Could you check a few things on this model? Use its own coordinates, in mm. A direction names the side the tool comes from. Coordinates: 2 decimals unless noted, no trailing zeros. Write each loop counter-clockwise with the first axis right and the second up, starting at its lowest first coordinate (ties: lowest second). Pieces come first, ordered by that corner, then holes. Notation, with made-up numbers: M 47.5,13 L 84.5,13 A19 cw 84.5,41 Z; hole C 81.25,-7 d3. An arc over 180 degrees is marked long. Write item = value, one per line.
```python
from build123d import *

# Parameters (mm, degrees)
ESBO_O1_W                = 100
ESBO_O1_H                = 95
RESSALTO_EXTRUS_O1_DEPTH = 1.5
ESBO_O2_R                = 1.5
ESBO_O2_W                = 40
ESBO_O2_H                = 3
CORTE_EXTRUS_O1_DEPTH    = 4
ESBO_O3_W                = 3
ESBO_O3_H                = 32
RESSALTO_EXTRUS_O2_DEPTH = 3
CUT_EXTRUDE1_DEPTH       = 1
CUT_EXTRUDE1_DEPTH_BACK  = 4
CUT_EXTRUDE4_DEPTH       = 2.5
CUT_EXTRUDE4_DEPTH_BACK  = 2.5
FILLET1_R                = 5
SKETCH3_W                = 3
SKETCH3_H                = 30
SKETCH3_H_2              = 17
SKETCH3_W_2              = 8
SKETCH3_H_3              = 3
CUT_EXTRUDE5_DEPTH       = 2.5
CUT_EXTRUDE5_DEPTH_BACK  = 2.5
SKETCH4_R                = 1.1
SKETCH4_W                = 12.2
SKETCH4_H                = 22.5
CUT_EXTRUDE6_DEPTH       = 1
CUT_EXTRUDE6_DEPTH_BACK  = 4


with BuildPart() as part:
    # Esboço1 → Ressalto-extrusão1 (new body, symmetric)
    with BuildSketch(Plane.XY):
        Rectangle(ESBO_O1_W, ESBO_O1_H)
    extrude(amount=RESSALTO_EXTRUS_O1_DEPTH, both=True)

    # Esboço2 → Corte-extrusão1 (cut, through all)
    with BuildSketch(Plane.XY.offset(1.5)):
        with Locations((-33, -1)):
            Circle(ESBO_O2_R)
        with Locations((33, -1)):
            Circle(ESBO_O2_R)
        with Locations((0, -46)):
            Rectangle(ESBO_O2_W, ESBO_O2_H)
        with Locations((0, -1)):
            Rectangle(ESBO_O2_W, ESBO_O2_H)
    extrude(amount=-CORTE_EXTRUS_O1_DEPTH, mode=Mode.SUBTRACT)

    # Esboço3 → Ressalto-extrusão2 (add, through all)
    with BuildSketch(Plane.XY.offset(1.5)):
        with Locations((-51.5, -31.5)):
            Rectangle(ESBO_O3_W, ESBO_O3_H)
        with Locations((51.5, -31.5)):
            Rectangle(ESBO_O3_W, ESBO_O3_H)
        with Locations((-51.5, 31.5)):
            Rectangle(ESBO_O3_W, ESBO_O3_H)
        with Locations((51.5, 31.5)):
            Rectangle(ESBO_O3_W, ESBO_O3_H)
    extrude(amount=-RESSALTO_EXTRUS_O2_DEPTH)

    # Sketch1 → Cut-Extrude1 (cut, two sides)
    with BuildSketch(Plane(origin=(0, 0, -1.5), x_dir=(-1, 0, 0), z_dir=(0, 0, -1))) as cut_extrude1_sk:
        with BuildLine():
            Line((-36.5, 39.75), (-36.5, 26.75))
            ThreePointArc((-36.5, 26.75), (-36.939339828, 25.689339828), (-38, 25.25))
            Line((-38, 25.25), (-41, 25.25))
            ThreePointArc((-41, 25.25), (-42.060660172, 24.810660172), (-42.5, 23.75))
            Line((-42.5, 23.75), (-42.5, 23.5))
            ThreePointArc((-42.5, 23.5), (-44, 22), (-45.5, 23.5))
            Line((-45.5, 23.5), (-45.5, 23.75))
            ThreePointArc((-45.5, 23.75), (-45.74500996, 24.571583836), (-46.4, 25.124772708))
            ThreePointArc((-46.4, 25.124772708), (-46.836660027, 25.49356529), (-47, 26.041287847))
            Line((-47, 26.041287847), (-47, 40.458712153))
            ThreePointArc((-47, 40.458712153), (-46.836660027, 41.00643471), (-46.4, 41.375227292))
            ThreePointArc((-46.4, 41.375227292), (-45.74500996, 41.928416164), (-45.5, 42.75))
            Line((-45.5, 42.75), (-45.5, 43))
            ThreePointArc((-45.5, 43), (-44, 44.5), (-42.5, 43))
            Line((-42.5, 43), (-42.5, 42.75))
            ThreePointArc((-42.5, 42.75), (-42.060660172, 41.689339828), (-41, 41.25))
            Line((-41, 41.25), (-38, 41.25))
            ThreePointArc((-38, 41.25), (-36.939339828, 40.810660172), (-36.5, 39.75))
        make_face()
        with BuildLine():
            Line((47, 40.458712153), (47, 26.041287847))
            ThreePointArc((47, 26.041287847), (46.836660027, 25.49356529), (46.4, 25.124772708))
            ThreePointArc((46.4, 25.124772708), (45.74500996, 24.571583836), (45.5, 23.75))
            Line((45.5, 23.75), (45.5, 23.5))
            ThreePointArc((45.5, 23.5), (44, 22), (42.5, 23.5))
            Line((42.5, 23.5), (42.5, 23.75))
            ThreePointArc((42.5, 23.75), (42.060660172, 24.810660172), (41, 25.25))
            Line((41, 25.25), (38, 25.25))
            ThreePointArc((38, 25.25), (36.939339828, 25.689339828), (36.5, 26.75))
            Line((36.5, 26.75), (36.5, 39.75))
            ThreePointArc((36.5, 39.75), (36.939339828, 40.810660172), (38, 41.25))
            Line((38, 41.25), (41, 41.25))
            ThreePointArc((41, 41.25), (42.060660172, 41.689339828), (42.5, 42.75))
            Line((42.5, 42.75), (42.5, 43))
            ThreePointArc((42.5, 43), (44, 44.5), (45.5, 43))
            Line((45.5, 43), (45.5, 42.75))
            ThreePointArc((45.5, 42.75), (45.74500996, 41.928416164), (46.4, 41.375227292))
            ThreePointArc((46.4, 41.375227292), (46.836660027, 41.00643471), (47, 40.458712153))
        make_face()
    extrude(amount=CUT_EXTRUDE1_DEPTH, mode=Mode.SUBTRACT)
    extrude(cut_extrude1_sk.sketch, amount=-CUT_EXTRUDE1_DEPTH_BACK, mode=Mode.SUBTRACT)

    # Sketch2 → Cut-Extrude4 (cut, two sides)
    with BuildSketch(Plane.XY) as cut_extrude4_sk:
        with BuildLine():
            Line((-0.5, -32.5), (0.5, -32.5))
            ThreePointArc((0.5, -32.5), (1.207106781, -32.792893219), (1.5, -33.5))
            Line((1.5, -33.5), (1.5, -38.23))
            Line((1.5, -38.23), (2.85, -38.23))
            Line((2.85, -38.23), (2.85, -40.5))
            Line((2.85, -40.5), (1.5, -40.5))
            Line((1.5, -40.5), (1.5, -44.5))
            Line((1.5, -44.5), (-1.5, -44.5))
            Line((-1.5, -44.5), (-1.5, -40.5))
            Line((-1.5, -40.5), (-2.85, -40.5))
            Line((-2.85, -40.5), (-2.85, -38.23))
            Line((-2.85, -38.23), (-1.5, -38.23))
            Line((-1.5, -38.23), (-1.5, -33.5))
            ThreePointArc((-1.5, -33.5), (-1.207106781, -32.792893219), (-0.5, -32.5))
        make_face()
    extrude(amount=CUT_EXTRUDE4_DEPTH, mode=Mode.SUBTRACT)
    extrude(cut_extrude4_sk.sketch, amount=-CUT_EXTRUDE4_DEPTH_BACK, mode=Mode.SUBTRACT)

    # Fillet1
    fillet1_edges = [part.edges().sort_by_distance(p)[0] for p in [
        (53, 47.5, 0),
        (-53, 47.5, 0),
    ]]
    fillet(fillet1_edges, radius=FILLET1_R)

    # Sketch3 → Cut-Extrude5 (cut, two sides)
    with BuildSketch(Plane.XY) as cut_extrude5_sk:
        with Locations((7.5, 29.5)):
            Rectangle(SKETCH3_W, SKETCH3_H)
        with Locations((7.5, -17)):
            Rectangle(SKETCH3_W, SKETCH3_H_2)
        with Locations((-7.5, 29.5)):
            Rectangle(SKETCH3_W, SKETCH3_H)
        with Locations((-1.5, -24)):
            Rectangle(SKETCH3_W_2, SKETCH3_H_3)
    extrude(amount=CUT_EXTRUDE5_DEPTH, mode=Mode.SUBTRACT)
    extrude(cut_extrude5_sk.sketch, amount=-CUT_EXTRUDE5_DEPTH_BACK, mode=Mode.SUBTRACT)

    # Sketch4 → Cut-Extrude6 (cut, two sides)
    with BuildSketch(Plane.XY.offset(1.5)) as cut_extrude6_sk:
        with Locations((20.9, 31.65)):
            Circle(SKETCH4_R)
        with Locations((20.9, 3.85)):
            Circle(SKETCH4_R)
        with Locations((20.9, 17.75)):
            Rectangle(SKETCH4_W, SKETCH4_H)
    extrude(amount=CUT_EXTRUDE6_DEPTH, mode=Mode.SUBTRACT)
    extrude(cut_extrude6_sk.sketch, amount=-CUT_EXTRUDE6_DEPTH_BACK, mode=Mode.SUBTRACT)


solid = part.part
```
Item 1: Imagine slicing it at A-A (y = 37). Write out the boundary of the cut face in (x, z), and give its area (3 significant figures).
Numbers:
outline = M -53,-1.5 L -47,-1.5 L -47,1.5 L -53,1.5 Z; M -36.5,-1.5 L -9,-1.5 L -9,1.5 L -36.5,1.5 Z; M -6,-1.5 L 6,-1.5 L 6,1.5 L -6,1.5 Z; M 9,-1.5 L 36.5,-1.5 L 36.5,1.5 L 9,1.5 Z; M 47,-1.5 L 53,-1.5 L 53,1.5 L 47,1.5 Z
area = 237 mm²
Item 2: Imagine slicing it at D-D (y = -20). Write out the boundary of the cut face in (x, z).
Numbers:
outline = M -53,-1.5 L 6,-1.5 L 6,1.5 L -53,1.5 Z; M 9,-1.5 L 53,-1.5 L 53,1.5 L 9,1.5 Z
Item 3: If I drill on line 1 along X through (y, z) = (34.5, 0.45); line 2 along Y through (x, z) = (-0.5, -0.35); line 3 along Y through (x, z) = (20.9, 0.6), over which ranges is the centre line in solid material (lowest first)?
Numbers:
line_1 = -53 to -47, -36.5 to -9, -6 to 6, 9 to 36.5, 47 to 53
line_2 = -32.5 to -25.5, -22.5 to -2.5, 0.5 to 47.5
line_3 = -47.5 to 2.75, 4.95 to 6.5, 29 to 30.55, 32.75 to 47.5
Item 4: I'm going to push flat-ended pins straight in: P1, Ø0.9, axis at x = 18.5, z = -0.5, coming from the -Y side; P2, Ø1.5, axis at y = 0.5, z = -1, coming from the -X side. Where does each tip first touch, or does it pass through?
Numbers:
P1 = -44.5
P2 = -50
Item 5: Imagine slicing it at C-C (y = -1). Write out the boundary of the cut face in (x, z), and give its area (3 significant figures).
Numbers:
outline = M -50,-1.5 L -34.5,-1.5 L -34.5,1.5 L -50,1.5 Z; M -31.5,-1.5 L -20,-1.5 L -20,1.5 L -31.5,1.5 Z; M 20,-1.5 L 31.5,-1.5 L 31.5,1.5 L 20,1.5 Z; M 34.5,-1.5 L 50,-1.5 L 50,1.5 L 34.5,1.5 Z
area = 162 mm²
Item 6: If we mould it in two halves opening along Y, with no side actions, what happens to faces 1 (the face through (-53, 29, 0)), 2 (the face through (51.57, 46, -0.02)), 3 (the face through (36, -47.5, 0)), 4 (the face through (-50, 0, 0))? For each: pulls with the +Y half, pulls with the -Y half, needs draft (parallel to the pull), parting line crosses it, or undercut.
Numbers:
face_1 = needs draft
face_2 = pulls with the +Y half
face_3 = pulls with the -Y half
face_4 = undercut
Item 7: For faces 5 (the face through (0, -2.5, 0)), 6 (the face through (-20, -46, 0)), 7 (the face through (-1, 47.5, 0)), 8 (the face through (51, 15.5, 0)), which set-ups out of +Z, -Z, +X, -X, +Y, -Y let a thin tool reach every point of the face, with its end or its side?
Numbers:
face_5 = +Z, -Z
face_6 = +Z, -Z, -Y
face_7 = +Z, -Z, +X, -X, +Y
face_8 = +Z, -Z, +X
Item 8: Imagine slicing it at B-B (x = -18). Write out the boundary of the cut face in (y, z).
Numbers:
outline = M -44.5,-1.5 L -2.5,-1.5 L -2.5,1.5 L -44.5,1.5 Z; M 0.5,-1.5 L 47.5,-1.5 L 47.5,1.5 L 0.5,1.5 Z
